Read the model definition and answer for the solid it produces. Units are mm, in the model's axes. A direction names the side the tool comes from. Give positions to 0.01 mm unless a question says otherwise; leave off trailing zeros. Loops run counter-clockwise (first coordinate to the right, second up) from the corner with the lowest first, then second, coordinate; pieces in that order, holes last. Notation, with made-up numbers: (62, -6.5) - (96, -6.5) arc R13 ccw to (96, -2.5) - close; hole circle Ø2 at (-24, 68). An arc over 180 degrees is marked (long way). Use a Markdown table: item, result. Add a question column.
Item 1: A cutting plane is placed at B-B (x = 0). Give the number of separate pieces and of enclosed holes in the cut face, plus the area to 3 significant figures.
Item 2: Each of these flat-tipped pins is pushed along its axis until it touches: P1, Ø1, axis at x = -1.5, z = 9, coming from the +Y side; P2, Ø2, axis at x = 2, y = 39, coming from the -Z side; P3, Ø5, axis at x = 0, z = 0, coming from the +Y side; P4, Ø8, axis at y = 11.5, z = 23.5, coming from the -X side. Where does it stop, or does it pass through?
Item 3: Which of the six approach directions +Z, -Z, +X, -X, +Y, -Y give full straight-line access (tool end or side, diameter ignored) to faces 4 (the face through (0, 34, 7)), 5 (the face through (1.3, 1, -1.3)), 6 (the face through (0, 4, 29))?
Item 4: For a pull along Y with two mould halves and no side action, classify faces 1 (the face through (0, 36, 9)), 2 (the face through (0, 0, 22)), 3 (the face through (1.615, 40.04, 17.331)) as +Y half, -Y half, draft (parallel to the pull), parting line (faces both ways), or undercut.
Item 5: Consider probe 1 along Y at (x, z) = (-2.75, 0.5); probe 2 along Z at (x, y) = (3.75, 2.5); probe 3 along Z at (x, y) = (-2.5, 23). Determine where each line is inside the solid, lowest interval first. Write a range as [from, to].
Item 6: A cutting plane is placed at A-A (z = 0). Determine the outline of the cut face in (x, y), plus the area to 3 significant figures.
from build123d import *

# Parameters (mm, degrees)
SKETCH1_W           = 10
SKETCH1_H           = 20
BOSS_EXTRUDE1_DEPTH = 3
SKETCH2_R           = 1.6
CUT_EXTRUDE1_DEPTH  = 4
SKETCH3_R           = 3.1
CUT_EXTRUDE2_DEPTH  = 1
SKETCH4_W           = 10
SKETCH4_H           = 43
BOSS_EXTRUDE2_DEPTH = 3
SKETCH5_W           = 10
SKETCH5_H           = 6
BOSS_EXTRUDE3_DEPTH = 3
CHAMFER1_SIZE       = 2.8
BOSS_EXTRUDE4_DEPTH = 10
SKETCH7_R           = 3.5
BOSS_EXTRUDE5_DEPTH = 2
SKETCH10_W          = 10
SKETCH10_H          = 3
CUT_EXTRUDE6_DEPTH  = 4
FILLET2_R           = 1
SKETCH8_R           = 1.5
CUT_EXTRUDE4_DEPTH  = 6


with BuildPart() as part:
    # Sketch1 → Boss-Extrude1 (new body)
    with BuildSketch(Plane(origin=(0, 0, 0), x_dir=(1, 0, 0), z_dir=(0, 1, 0))):
        Rectangle(SKETCH1_W, SKETCH1_H)
    extrude(amount=BOSS_EXTRUDE1_DEPTH)

    # Sketch2 → Cut-Extrude1 (cut, through all)
    with BuildSketch(Plane.XZ):
        Circle(SKETCH2_R)
    extrude(amount=-CUT_EXTRUDE1_DEPTH, mode=Mode.SUBTRACT)

    # Sketch3 → Cut-Extrude2 (cut)
    with BuildSketch(Plane.XZ):
        Circle(SKETCH3_R)
    extrude(amount=-CUT_EXTRUDE2_DEPTH, mode=Mode.SUBTRACT)

    # Sketch4 → Boss-Extrude2 (add)
    with BuildSketch(Plane.XY.offset(10)):
        with Locations((0, 21.5)):
            Rectangle(SKETCH4_W, SKETCH4_H)
    extrude(amount=BOSS_EXTRUDE2_DEPTH)

    # Sketch5 → Boss-Extrude3 (add)
    with BuildSketch(Plane(origin=(0, 0, 10), x_dir=(-1, 0, 0), z_dir=(0, 0, -1))):
        with Locations((0, 13)):
            Rectangle(SKETCH5_W, SKETCH5_H)
        with Locations((0, 33)):
            Rectangle(SKETCH5_W, SKETCH5_H)
    extrude(amount=BOSS_EXTRUDE3_DEPTH)

    # Chamfer1
    chamfer1_edges = [part.edges().sort_by_distance(p)[0] for p in [
        (0, 30, 7),
        (0, 10, 7),
    ]]
    chamfer(chamfer1_edges, length=CHAMFER1_SIZE)

    # Sketch6 → Boss-Extrude4 (add)
    with BuildSketch(Plane.ZY.offset(5)):
        Polygon((13, 40), (16, 40), (50.698703146, 4), (50.698703146, 0), (13, 0), (13, 4), (45.14314759, 4), (13, 37.348604079), align=None)
    extrude(amount=-BOSS_EXTRUDE4_DEPTH)

    # Sketch7 → Boss-Extrude5 (add)
    with BuildSketch(Plane(origin=(0, -24.3220742, 77.997015511), x_dir=(1, 0, 0), z_dir=(0, -0.693974063, -0.72))):
        with Locations((0, -43.336214167)):
            Circle(SKETCH7_R)
        with Locations((0, -85.336214167)):
            Circle(SKETCH7_R)
    extrude(amount=-BOSS_EXTRUDE5_DEPTH)

    # Sketch10 → Cut-Extrude6 (cut, through all)
    with BuildSketch(Plane(origin=(0, 3, 0), x_dir=(1, 0, 0), z_dir=(0, 1, 0))):
        with Locations((0, 8.5)):
            Rectangle(SKETCH10_W, SKETCH10_H)
    extrude(amount=-CUT_EXTRUDE6_DEPTH, mode=Mode.SUBTRACT)

    # Fillet2
    fillet2_edges = [part.edges().sort_by_distance(p)[0] for p in [
        (-5, 0, 21.849351573),
        (0, 0, -7),
        (0, 43, 13),
        (0, 36, 7),
        (5, 0, 21.849351573),
        (0, 16, 7),
        (0, 40, 13),
        (0, 40, 16),
        (0, 4, 50.698703146),
        (0, 0, 50.698703146),
        (-5, 2, 50.698703146),
        (-5, 22, 33.349351573),
        (5, 22, 33.349351573),
        (5, 2, 50.698703146),
    ]]
    fillet(fillet2_edges, radius=FILLET2_R)

    # Sketch8 → Cut-Extrude4 (cut)
    with BuildSketch(Plane(origin=(0, 28.646529331, 29.720853012), x_dir=(-1, 0, 0), z_dir=(0, 0.693974063, 0.72))):
        with Locations((0, 28.303585007)):
            Circle(SKETCH8_R)
        with Locations((0, -13.696414993)):
            Circle(SKETCH8_R)
    extrude(amount=-CUT_EXTRUDE4_DEPTH, mode=Mode.SUBTRACT)


solid = part.part
Geometry says:
| question | item | result |
|---|---|---|
| 1 | separate pieces | 3 |
| 1 | enclosed holes | 0 |
| 1 | area | 534 mm² |
| 2 | P1 | y = 36 |
| 2 | P2 | z = 10 |
| 2 | P3 | y = 3 |
| 2 | P4 | through |
| 3 | face 4 | -Z, +X, -X, +Y |
| 3 | face 5 | -Y |
| 3 | face 6 | +X, -X |
| 4 | face 1 | +Y half |
| 4 | face 2 | -Y half |
| 4 | face 3 | undercut |
| 5 | probe 1 | [1, 3] |
| 5 | probe 2 | [-7, 50.7] |
| 5 | probe 3 | [10, 13], [26.83, 32.39] |
| 6 | outline | (-5, 1) arc R1 ccw to (-4, 0) - (-3.1, 0) - (-3.1, 1) - (-1.6, 1) - (-1.6, 3) - (-5, 3) - close; (1.6, 1) - (3.1, 1) - (3.1, 0) - (4, 0) arc R1 ccw to (5, 1) - (5, 3) - (1.6, 3) - close |
| 6 | area | 17.0 mm² |
